Verification items for the finished model (mm, model axes). A direction names the side the tool comes from. Give positions to 0.01 mm unless a question says otherwise; leave off trailing zeros. Write each loop counter-clockwise with the first axis right and the second up, starting at its lowest first coordinate (ties: lowest second). Pieces come first, ordered by that corner, then holes.
from build123d import *

# Parameters (mm, degrees)
EXTRUDE_1_DEPTH     = 42
SKETCH_2_R          = 2
CUT_EXTRUDE_1_DEPTH = 65.899922958
SKETCH_3_R          = 2.25
CUT_EXTRUDE_2_DEPTH = 55
CUT_EXTRUDE_3_DEPTH = 5
SKETCH_5_R          = 3.5
CUT_EXTRUDE_4_DEPTH = 5
SKETCH_6_R          = 3.5
CUT_EXTRUDE_5_DEPTH = 5


with BuildPart() as part:
    # Sketch 1 → Extrude 1 (new body)
    with BuildSketch(Plane.XY):
        Polygon((12, 10), (-4, 10), (-4, -10), (12, -10), (12, -24), (-12, -24), (-12, 24), (12, 24), align=None)
    extrude(amount=EXTRUDE_1_DEPTH)

    # Sketch 2 → Cut-Extrude 1 (cut, through all)
    with BuildSketch(Plane(origin=(0, 24, 0), x_dir=(1, 0, 0), z_dir=(0, 1, 0))):
        with Locations(Location((2, -5, 0), (0, 0, 270))):
            Circle(SKETCH_2_R)
        with Locations(Location((2, -16, 0), (0, 0, 270))):
            Circle(SKETCH_2_R)
        with Locations(Location((2, -26, 0), (0, 0, 270))):
            Circle(SKETCH_2_R)
        with Locations(Location((2, -37, 0), (0, 0, 270))):
            Circle(SKETCH_2_R)
    extrude(amount=-CUT_EXTRUDE_1_DEPTH, mode=Mode.SUBTRACT)

    # Sketch 3 → Cut-Extrude 2 (cut, through all)
    with BuildSketch(Plane.ZY.offset(12)):
        with Locations(Location((10, 15, 0), (0, 0, 270))):
            Circle(SKETCH_3_R)
        with Locations(Location((32, 15, 0), (0, 0, 270))):
            Circle(SKETCH_3_R)
        with Locations(Location((32, -15, 0), (0, 0, 90))):
            Circle(SKETCH_3_R)
        with Locations(Location((10, -15, 0), (0, 0, 90))):
            Circle(SKETCH_3_R)
    extrude(amount=-CUT_EXTRUDE_2_DEPTH, mode=Mode.SUBTRACT)

    # Sketch 4 → Cut-Extrude 3 (cut)
    with BuildSketch(Plane(origin=(12, 0, 0), x_dir=(0, 0, -1), z_dir=(1, 0, 0))):
        Polygon((-5.843078062, 15), (-7.921539031, 18.6), (-12.078460969, 18.6), (-14.156921938, 15), (-12.078460969, 11.4), (-7.921539031, 11.4), align=None)
        Polygon((-27.843078062, 15), (-29.921539031, 18.6), (-34.078460969, 18.6), (-36.156921938, 15), (-34.078460969, 11.4), (-29.921539031, 11.4), align=None)
        Polygon((-27.843078062, -15), (-29.921539031, -11.4), (-34.078460969, -11.4), (-36.156921938, -15), (-34.078460969, -18.6), (-29.921539031, -18.6), align=None)
        Polygon((-5.843078062, -15), (-7.921539031, -11.4), (-12.078460969, -11.4), (-14.156921938, -15), (-12.078460969, -18.6), (-7.921539031, -18.6), align=None)
    extrude(amount=-CUT_EXTRUDE_3_DEPTH, mode=Mode.SUBTRACT)

    # Sketch 5 → Cut-Extrude 4 (cut)
    with BuildSketch(Plane.XZ.offset(24)):
        with Locations(Location((2, 16, 0), (0, 0, 270))):
            Circle(SKETCH_5_R)
        with Locations(Location((2, 37, 0), (0, 0, 270))):
            Circle(SKETCH_5_R)
        Polygon((2, 21.843078062), (5.6, 23.921539031), (5.6, 28.078460969), (2, 30.156921938), (-1.6, 28.078460969), (-1.6, 23.921539031), align=None)
        Polygon((6.156921938, 5), (4.078460969, 8.6), (-0.078460969, 8.6), (-2.156921938, 5), (-0.078460969, 1.4), (4.078460969, 1.4), align=None)
    extrude(amount=-CUT_EXTRUDE_4_DEPTH, mode=Mode.SUBTRACT)

    # Sketch 6 → Cut-Extrude 5 (cut)
    with BuildSketch(Plane(origin=(0, 24, 0), x_dir=(1, 0, 0), z_dir=(0, 1, 0))):
        with Locations(Location((2, -26, 0), (0, 0, 270))):
            Circle(SKETCH_6_R)
        with Locations(Location((2, -5, 0), (0, 0, 270))):
            Circle(SKETCH_6_R)
        Polygon((2, -11.843078062), (-1.6, -13.921539031), (-1.6, -18.078460969), (2, -20.156921938), (5.6, -18.078460969), (5.6, -13.921539031), align=None)
        Polygon((2, -32.843078062), (-1.6, -34.921539031), (-1.6, -39.078460969), (2, -41.156921938), (5.6, -39.078460969), (5.6, -34.921539031), align=None)
    extrude(amount=-CUT_EXTRUDE_5_DEPTH, mode=Mode.SUBTRACT)


solid = part.part
Item 1: Set-up check for faces 1 (the face through (-2.633, -13.79, 8.103)), 2 (the face through (-1.6, 22, 37)), 3 (the face through (-5, 0, 42)), 4 (the face through (10, 13, 29)), 5 (the face through (-1, -22, 3)): record each of +Z, -Z, +X, -X, +Y, -Y from which the full face is reachable in a straight line by a thin tool's end or side.
Answer key:
face 1: +X, -X
face 2: +Y
face 3: +Z, +X, -X, +Y, -Y
face 4: +X
face 5: -Y
Item 2: Sectioned sample at B-B on x = -7. Record the cut outline in (y, z).
Answer key:
outline: (-24, 0) - (24, 0) - (24, 42) - (-24, 42) - close; hole circle Ø4.5 at (-15, 10); hole circle Ø4.5 at (-15, 32); hole circle Ø4.5 at (15, 10); hole circle Ø4.5 at (15, 32)
Item 3: Sectioned sample at A-A on z = 10. Record the cut outline in (x, y).
Answer key:
outline: (-12, -24) - (12, -24) - (12, -18.6) - (7, -18.6) - (7, -17.25) - (-12, -17.25) - close; (-12, -12.75) - (7, -12.75) - (7, -11.4) - (12, -11.4) - (12, -10) - (-4, -10) - (-4, 10) - (12, 10) - (12, 11.4) - (7, 11.4) - (7, 12.75) - (-12, 12.75) - close; (-12, 17.25) - (7, 17.25) - (7, 18.6) - (12, 18.6) - (12, 24) - (-12, 24) - close
Item 4: Scan lines: line 1 along Y through (x, z) = (11, 37.5); line 2 along X through (y, z) = (-21, 37); line 3 along Y through (x, z) = (-1.25, 8). Record each from-to range of solid material in increasing order.
Answer key:
line 1: y = -24 to -10, 10 to 24
line 2: x = -12 to -1.5, 5.5 to 12
line 3: y = -24 to -16.03, -13.97 to -10, 10 to 13.97, 16.03 to 24
Item 5: Depth check by flat-ended pin: pin 1 (6 mm diameter, centred on x = 1, z = 16, fed in from +Y); pin 2 (4 mm diameter, centred on y = -15, z = 10, fed in from +X); pin 3 (5 mm diameter, centred on y = 0.5, z = 17.5, fed in from +X); pin 4 (5.5 mm diameter, centred on x = 2, z = 5, fed in from -Y). Enter the tip coordinate at first touch or a pass-through.
Answer key:
pin 1: stops at y = 24
pin 2: passes through
pin 3: stops at x = -4
pin 4: stops at y = -19
Item 6: Sectioned sample at D-D on z = 16. Record the cut outline in (x, y).
Answer key:
outline: (-12, -24) - (-1.5, -24) - (-1.5, -19) - (0, -19) - (0, -10) - (-4, -10) - (-4, 10) - (0, 10) - (0, 19) - (-1.6, 19) - (-1.6, 24) - (-12, 24) - close; (4, -19) - (5.5, -19) - (5.5, -24) - (12, -24) - (12, -10) - (4, -10) - close; (4, 10) - (12, 10) - (12, 24) - (5.6, 24) - (5.6, 19) - (4, 19) - close
Item 7: Release check for a two-part mould opening along X. For faces 6 (the face through (10, -17, 35)), 7 (the face through (7, -17, 30)), 8 (the face through (0.226, -14.437, 16.923)), 9 (the face through (0.8, 14.6, 3.4)) record: released by +X, released by -X, zero draft, split by the parting line, or undercut.
Answer key:
face 6: zero draft
face 7: released by +X
face 8: undercut
face 9: undercut
Item 8: Sectioned sample at C-C on y = -8.5. Record the cut outline in (x, z), then the cut area to 3 significant figures.
Answer key:
outline: (-12, 0) - (-4, 0) - (-4, 42) - (-12, 42) - close
area: 336 mm2
